```python
from build123d import *

# Parameters (mm, degrees)
SKETCH_1_W                       = 75
SKETCH_1_H                       = 192
SM_BASE_FLANGE_2_DEPTH           = 3
SM_EDGE_FLANGE_1_STRIP_W         = 18
SM_EDGE_FLANGE_1_STRIP_H         = 3
SM_EDGE_FLANGE_1_STRIP_CUT_DEPTH = 75
SM_EDGE_FLANGE_1_DEPTH           = 75
SM_EDGE_FLANGE_2_DEPTH           = 75
SKETCH_18_W                      = 3
SKETCH_18_H                      = 30
SKETCH_18_H_2                    = 61
CUT_EXTRUDE_1_DEPTH              = 30
SKETCH_19_W                      = 20
SKETCH_19_H                      = 3
CUT_EXTRUDE_2_DEPTH              = 203
SKETCH_20_R                      = 1
CUT_EXTRUDE_3_DEPTH              = 3


# Sheet-metal steps are written as plain solids
with BuildPart() as part:
    # 草图1 → 基体-法兰2 (new body)
    with BuildSketch(Plane.XY):
        with Locations((27.011429417, -3.544407938)):
            Rectangle(SKETCH_1_W, SKETCH_1_H)
    extrude(amount=-SM_BASE_FLANGE_2_DEPTH)

    # 边线-法兰1 strip (across the edge) → 边线-法兰1 strip cut (cut)
    with BuildSketch(Plane(origin=(64.511429417, -99.544407938, -3), x_dir=(0, 1, 0), z_dir=(-1, 0, 0))):
        with Locations((-6, -1.5)):
            Rectangle(SM_EDGE_FLANGE_1_STRIP_W, SM_EDGE_FLANGE_1_STRIP_H)
    extrude(amount=SM_EDGE_FLANGE_1_STRIP_CUT_DEPTH, mode=Mode.SUBTRACT)

    # 边线-法兰1 section (across the edge) → 边线-法兰1 (add)
    with BuildSketch(Plane(origin=(64.511429417, -99.544407938, -3), x_dir=(0, 1, 0), z_dir=(-1, 0, 0))):
        with BuildLine():
            Line((-3, 3), (-3, 20))
            Line((-3, 20), (0, 20))
            Line((0, 20), (0, 3))
            ThreePointArc((0, 3), (0.878679656, 0.878679656), (3, 0))
            Line((3, 0), (3, -3))
            ThreePointArc((3, -3), (-1.242640687, -1.242640687), (-3, 3))
        make_face()
    extrude(amount=SM_EDGE_FLANGE_1_DEPTH)

    # 边线-法兰2 section (across the edge) → 边线-法兰2 (add)
    with BuildSketch(Plane(origin=(-10.488570583, 95.455592062, -3), x_dir=(0, -1, 0), z_dir=(1, 0, 0))):
        with BuildLine():
            Line((-3, 3), (-3, 20))
            Line((-3, 20), (0, 20))
            Line((0, 20), (0, 3))
            ThreePointArc((0, 3), (0.878679656, 0.878679656), (3, 0))
            Line((3, 0), (3, -3))
            ThreePointArc((3, -3), (-1.242640687, -1.242640687), (-3, 3))
        make_face()
    extrude(amount=SM_EDGE_FLANGE_2_DEPTH)

    # 草图18 → 切除-拉伸1 (cut)
    with BuildSketch(Plane.XY):
        with Locations((63.011429417, -87.544407938)):
            Rectangle(SKETCH_18_W, SKETCH_18_H)
        with Locations((63.011429417, 83.455592062)):
            Rectangle(SKETCH_18_W, SKETCH_18_H)
        with Locations((63.011429417, -2.044407938)):
            Rectangle(SKETCH_18_W, SKETCH_18_H_2)
        with Locations((-8.988570583, -2.044407938)):
            Rectangle(SKETCH_18_W, SKETCH_18_H_2)
        with Locations((-8.988570583, -87.544407938)):
            Rectangle(SKETCH_18_W, SKETCH_18_H)
        with Locations((-8.988570583, 83.455592062)):
            Rectangle(SKETCH_18_W, SKETCH_18_H)
    extrude(amount=-CUT_EXTRUDE_1_DEPTH, mode=Mode.SUBTRACT)

    # 草图19 → 切除-拉伸2 (cut)
    with BuildSketch(Plane.XZ.offset(102.544407938)):
        with Locations((2.511429417, -21.5)):
            Rectangle(SKETCH_19_W, SKETCH_19_H)
        with Locations((51.511429417, -21.5)):
            Rectangle(SKETCH_19_W, SKETCH_19_H)
    extrude(amount=-CUT_EXTRUDE_2_DEPTH, mode=Mode.SUBTRACT)

    # 草图20 → 切除-拉伸3 (cut)
    with BuildSketch(Plane.XY):
        with Locations((23.610533211, -47.310308186)):
            Circle(SKETCH_20_R)
        with Locations((28.610533211, -47.310308186)):
            Circle(SKETCH_20_R)
        with Locations((33.610533211, -47.310308186)):
            Circle(SKETCH_20_R)
        with Locations((38.610533211, -47.310308186)):
            Circle(SKETCH_20_R)
        with Locations((43.610533211, -47.310308186)):
            Circle(SKETCH_20_R)
        with Locations((28.610533211, -42.310308186)):
            Circle(SKETCH_20_R)
        with Locations((33.610533211, -42.310308186)):
            Circle(SKETCH_20_R)
        with Locations((38.610533211, -42.310308186)):
            Circle(SKETCH_20_R)
        with Locations((43.610533211, -42.310308186)):
            Circle(SKETCH_20_R)
        with Locations((28.610533211, -37.310308186)):
            Circle(SKETCH_20_R)
        with Locations((33.610533211, -37.310308186)):
            Circle(SKETCH_20_R)
        with Locations((38.610533211, -37.310308186)):
            Circle(SKETCH_20_R)
        with Locations((43.610533211, -37.310308186)):
            Circle(SKETCH_20_R)
        with Locations((28.610533211, -32.310308186)):
            Circle(SKETCH_20_R)
        with Locations((33.610533211, -32.310308186)):
            Circle(SKETCH_20_R)
        with Locations((38.610533211, -32.310308186)):
            Circle(SKETCH_20_R)
        with Locations((43.610533211, -32.310308186)):
            Circle(SKETCH_20_R)
        with Locations((28.610533211, -27.310308186)):
            Circle(SKETCH_20_R)
        with Locations((33.610533211, -27.310308186)):
            Circle(SKETCH_20_R)
        with Locations((38.610533211, -27.310308186)):
            Circle(SKETCH_20_R)
        with Locations((43.610533211, -27.310308186)):
            Circle(SKETCH_20_R)
        with Locations((28.610533211, -22.310308186)):
            Circle(SKETCH_20_R)
        with Locations((33.610533211, -22.310308186)):
            Circle(SKETCH_20_R)
        with Locations((38.610533211, -22.310308186)):
            Circle(SKETCH_20_R)
        with Locations((43.610533211, -22.310308186)):
            Circle(SKETCH_20_R)
        with Locations((28.610533211, -17.310308186)):
            Circle(SKETCH_20_R)
        with Locations((33.610533211, -17.310308186)):
            Circle(SKETCH_20_R)
        with Locations((38.610533211, -17.310308186)):
            Circle(SKETCH_20_R)
        with Locations((43.610533211, -17.310308186)):
            Circle(SKETCH_20_R)
        with Locations((28.610533211, -12.310308186)):
            Circle(SKETCH_20_R)
        with Locations((33.610533211, -12.310308186)):
            Circle(SKETCH_20_R)
        with Locations((38.610533211, -12.310308186)):
            Circle(SKETCH_20_R)
        with Locations((43.610533211, -12.310308186)):
            Circle(SKETCH_20_R)
        with Locations((23.610533211, -42.310308186)):
            Circle(SKETCH_20_R)
        with Locations((23.610533211, -37.310308186)):
            Circle(SKETCH_20_R)
        with Locations((23.610533211, -32.310308186)):
            Circle(SKETCH_20_R)
        with Locations((23.610533211, -27.310308186)):
            Circle(SKETCH_20_R)
        with Locations((23.610533211, -22.310308186)):
            Circle(SKETCH_20_R)
        with Locations((23.610533211, -17.310308186)):
            Circle(SKETCH_20_R)
        with Locations((23.610533211, -12.310308186)):
            Circle(SKETCH_20_R)
    extrude(amount=-CUT_EXTRUDE_3_DEPTH, mode=Mode.SUBTRACT)


solid = part.part
```
Input: part model. Units: mm. Frame: model coordinates. A direction names the side the tool comes from. Round coordinates to 2 decimals unless told otherwise and drop trailing zeros. Loops run counter-clockwise (first coordinate to the right, second up) from the corner with the lowest first, then second, coordinate; pieces in that order, holes last.
1) Set-up query: faces 5 (the flat face through (27, 95.456, -13)), 6 (the flat face through (-7.489, -94.3, -2.5)), 7 (the flat face through (61.511, -94.3, -2.5)), 8 (the flat face through (61.511, 86.7, -2.5)). Return all of +Z, -Z, +X, -X, +Y, -Y with unobstructed straight access to the full face (end or side cutting, diameter ignored); none if empty.
Ans:
face 5: -Z, +X, -X
face 6: +Z, -Z, -X, -Y
face 7: +Z, -Z, +X, -Y
face 8: +Z, -Z, +X, +Y
2) Section query A-A on z = -9. Return the cut outline in (x, y), plus the area to 3 significant figures.
Ans:
outline: (-7.49, -102.54) - (61.51, -102.54) - (61.51, -99.54) - (-7.49, -99.54) - close; (-7.49, 95.46) - (61.51, 95.46) - (61.51, 98.46) - (-7.49, 98.46) - close
area: 414 mm2
3) Pin query (flat end, axial travel): pin 1 (3.5 mm diameter, centred on x = 63.5, z = -1, fed in from -Y); pin 2 (2.5 mm diameter, centred on x = -9, z = -2, fed in from +Y); pin 3 (2.5 mm diameter, centred on x = 43.61, y = -27.31, fed in from -Z). Return the tip coordinate at first contact, or that it passes through.
Ans:
pin 1: stops at y = -72.54
pin 2: stops at y = 68.46
pin 3: stops at z = -3
4) Pull-direction query (Y, two-part tool) for faces 1 (the flat face through (26, -1, -3)), 2 (the flat face through (-7.489, 86.7, -2.5)), 3 (the flat face through (27, -102.544, -12)), 4 (the flat face through (27, 98.456, -12)); classes: released by +Y, released by -Y, zero draft, split by the parting line, or undercut.
Ans:
face 1: undercut
face 2: zero draft
face 3: released by -Y
face 4: released by +Y
5) Section query C-C on y = -6.5. Return the cut outline in (x, z).
Ans:
outline: (-7.49, -3) - (61.51, -3) - (61.51, 0) - (-7.49, 0) - close
6) Section query B-B on x = 50. Return the cut outline in (y, z), plus the area to 3 significant figures.
Ans:
outline: (-102.54, -20) - (-99.54, -20) - (-99.54, -6) arc R3 cw to (-96.54, -3) - (92.46, -3) arc R3 cw to (95.46, -6) - (95.46, -20) - (98.46, -20) - (98.46, -6) arc R6 ccw to (92.46, 0) - (-96.54, 0) arc R6 ccw to (-102.54, -6) - close
area: 693 mm2
7) Material intervals for line 1 (Y direction, x = 57, z = -19.5); line 2 (Z direction, x = 44.5, y = -39); line 3 (Y direction, x = 4, z = -5), sorted ascending.
Ans:
line 1: y = -102.54 to -99.54, 95.46 to 98.46
line 2: z = -3 to 0
line 3: y = -102.46 to -99.37, 95.28 to 98.37
8) Section query D-D on y = -55.5. Return the cut outline in (x, z), plus the area to 3 significant figures.
Ans:
outline: (-10.49, -3) - (64.51, -3) - (64.51, 0) - (-10.49, 0) - close
area: 225 mm2
